Geometry check sheet. Reference: the model listing, model coordinates, mm. A direction names the side the tool comes from. Round coordinates to 2 decimals unless told otherwise and drop trailing zeros. Write each loop counter-clockwise with the first axis right and the second up, starting at its lowest first coordinate (ties: lowest second). Pieces come first, ordered by that corner, then holes. Notation, with made-up numbers: M -22.5,-30 L 14.5,-30 A20 ccw 14.5,-25 Z; hole C -21.75,74.25 d4. An arc over 180 degrees is marked long. Use a Markdown table: item, result.
```python
from build123d import *

# Parameters (mm, degrees)
BOSS_EXTRUDE1_DEPTH = 1.651
SKETCH3_W           = 2.54
SKETCH3_H           = 1.694812446
SKETCH3_W_2         = 1.694812446
SKETCH3_H_2         = 2.54
BOSS_EXTRUDE2_DEPTH = 3.683
BOSS_EXTRUDE3_DEPTH = 1.27
BOSS_EXTRUDE4_DEPTH = 1.27
FILLET1_R           = 1.27
CHAMFER1_SIZE       = 0.508
FILLET2_R           = 0.254


with BuildPart() as part:
    # Sketch1 → Boss-Extrude1 (new body)
    with BuildSketch(Plane(origin=(0, 0, 0), x_dir=(1, 0, 0), z_dir=(0, 1, 0))):
        with BuildLine():
            Line((-7.62, 7.112), (-7.62, -7.112))
            ThreePointArc((-7.62, -7.112), (-7.471210245, -7.471210245), (-7.112, -7.62))
            Line((-7.112, -7.62), (7.112, -7.62))
            ThreePointArc((7.112, -7.62), (7.471210245, -7.471210245), (7.62, -7.112))
            Line((7.62, -7.112), (7.62, 7.112))
            ThreePointArc((7.62, 7.112), (7.471210245, 7.471210245), (7.112, 7.62))
            Line((7.112, 7.62), (-7.112, 7.62))
            ThreePointArc((-7.112, 7.62), (-7.471210245, 7.471210245), (-7.62, 7.112))
        make_face()
    extrude(amount=BOSS_EXTRUDE1_DEPTH)

    # Sketch3 → Boss-Extrude2 (add)
    with BuildSketch(Plane(origin=(0, 1.651, 0), x_dir=(1, 0, 0), z_dir=(0, 1, 0))):
        with Locations((0, 3.013059552)):
            Rectangle(SKETCH3_W, SKETCH3_H)
        with Locations((3.013059552, 0)):
            Rectangle(SKETCH3_W_2, SKETCH3_H_2)
        with Locations((0, -3.013059552)):
            Rectangle(SKETCH3_W, SKETCH3_H)
        with Locations((-3.013059552, 0)):
            Rectangle(SKETCH3_W_2, SKETCH3_H_2)
    extrude(amount=BOSS_EXTRUDE2_DEPTH)

    # Sketch4 → Boss-Extrude3 (add, symmetric)
    with BuildSketch(Plane.XY):
        with BuildLine():
            Line((-3.860465775, 5.334), (-4.251394799, 4.259931334))
            ThreePointArc((-4.251394799, 4.259931334), (-4.201247752, 3.879026697), (-3.860465775, 3.701626828))
            Line((-3.860465775, 3.701626828), (-3.860465775, 5.334))
        make_face()
        with BuildLine():
            Line((3.860465775, 5.334), (4.251394799, 4.259931334))
            ThreePointArc((4.251394799, 4.259931334), (4.201247752, 3.879026697), (3.860465775, 3.701626828))
            Line((3.860465775, 3.701626828), (3.860465775, 5.334))
        make_face()
    extrude(amount=BOSS_EXTRUDE3_DEPTH, both=True)

    # Sketch5 → Boss-Extrude4 (add, symmetric)
    with BuildSketch(Plane(origin=(0, 0, 0), x_dir=(0, 0, -1), z_dir=(1, 0, 0))):
        with BuildLine():
            Line((-3.860465775, 5.334), (-4.251394799, 4.259931334))
            ThreePointArc((-4.251394799, 4.259931334), (-4.201512131, 3.878082751), (-3.860465775, 3.699242027))
            Line((-3.860465775, 3.699242027), (-3.860465775, 5.334))
        make_face()
        with BuildLine():
            Line((3.860465775, 5.334), (4.251394799, 4.259931334))
            ThreePointArc((4.251394799, 4.259931334), (4.201512131, 3.878082751), (3.860465775, 3.699242027))
            Line((3.860465775, 3.699242027), (3.860465775, 5.334))
        make_face()
    extrude(amount=BOSS_EXTRUDE4_DEPTH, both=True)

    # Fillet1
    fillet1_edges = [part.edges().sort_by_distance(p)[0] for p in [
        (0, 5.334, -3.860465775),
        (3.860465775, 5.334, 0),
        (0, 5.334, 3.860465775),
        (-3.860465775, 5.334, 0),
    ]]
    fillet(fillet1_edges, radius=FILLET1_R)

    # Chamfer1
    chamfer1_edges = [part.edges().sort_by_distance(p)[0] for p in [
        (7.471210245, 1.651, 7.471210245),
        (7.62, 1.651, 0),
        (7.471210245, 1.651, -7.471210245),
        (0, 1.651, -7.62),
        (-7.471210245, 1.651, -7.471210245),
        (-7.62, 1.651, 0),
        (-7.471210245, 1.651, 7.471210245),
        (0, 1.651, 7.62),
    ]]
    chamfer(chamfer1_edges, length=CHAMFER1_SIZE - 0.0001)  # a hair under: the kernel refuses the full size

    # Fillet2
    fillet2_edges = [part.edges().sort_by_distance(p)[0] for p in [
        (0, 0, 7.62),
        (-7.471210245, 0, 7.471210245),
        (-7.62, 0, 0),
        (-7.471210245, 0, -7.471210245),
        (0, 0, -7.62),
        (7.471210245, 0, -7.471210245),
        (7.62, 0, 0),
        (7.471210245, 0, 7.471210245),
    ]]
    fillet(fillet2_edges, radius=FILLET2_R)


solid = part.part
```
Item 1: Cross-section at B-B, the plane y = 2.5. Record the cut outline in (x, z), and give its area (3 significant figures).
Outcome:
| item | result |
|---|---|
| outline | M -3.86,-1.27 L -2.17,-1.27 L -2.17,1.27 L -3.86,1.27 Z; M -1.27,-3.86 L 1.27,-3.86 L 1.27,-2.17 L -1.27,-2.17 Z; M -1.27,2.17 L 1.27,2.17 L 1.27,3.86 L -1.27,3.86 Z; M 2.17,-1.27 L 3.86,-1.27 L 3.86,1.27 L 2.17,1.27 Z |
| area | 17.2 mm2 |
Item 2: Go/stop test with flat-tipped pins: pin 1 (1.7 mm diameter, centred on y = 3, z = -3.5, fed in from +X); pin 2 (3 mm diameter, centred on y = 4, z = -0.5, fed in from -X); pin 3 (0.8 mm diameter, centred on y = 3.5, z = 0, fed in from +X) (3 decimals); pin 4 (2 mm diameter, centred on x = 2, z = -5.5, fed in from -Y). Record where each tip stops, or that it passes through.
Outcome:
| item | result |
|---|---|
| pin 1 | stops at x = 1.27 |
| pin 2 | stops at x = -4.28 |
| pin 3 | stops at x = 4.215 |
| pin 4 | stops at y = 0 |
Item 3: Access from +Z, -Z, +X, -X, +Y, -Y to the whole of each face (thin tool, end or side, straight path). Record for faces 1 (the face through (0, 3, -3.86)), 2 (the face through (3, 4, 1.27)), 3 (the face through (3, 4, -1.27)).
Outcome:
| item | result |
|---|---|
| face 1 | -Z, +X, -X |
| face 2 | +Z, +X, -X, +Y |
| face 3 | -Z, +X, -X, +Y |
Item 4: Mould release check, pull along Y, two halves, no side actions. Record for faces 4 (the face through (0, 3, 2.166)), 5 (the face through (0, 5.334, 2.6)), 6 (the face through (0, 3, 3.86)): +Y half, -Y half, draft (parallel to the pull), parting line (faces both ways), or undercut.
Outcome:
| item | result |
|---|---|
| face 4 | draft |
| face 5 | +Y half |
| face 6 | undercut |
Item 5: Material ranges on line 1 along X through (y, z) = (2.05, -0.25); line 2 along Z through (x, y) = (-1, 4.25); line 3 along Y through (x, z) = (-5.25, -5.5), recorded low to high. Write a range as from..to.
Outcome:
| item | result |
|---|---|
| line 1 | x = -3.86..-2.17, 2.17..3.86 |
| line 2 | z = -4.25..-2.17, 2.17..4.25 |
| line 3 | y = 0..1.65 |
Item 6: Cross-section at C-C, the plane z = 1.5. Record the cut outline in (x, y), and give its area (3 significant figures).
Outcome:
| item | result |
|---|---|
| outline | M -7.62,0.25 A0.25 ccw -7.37,0 L 7.37,0 A0.25 ccw 7.62,0.25 L 7.62,1.14 L 7.11,1.65 L -7.11,1.65 L -7.62,1.14 Z |
| area | 24.9 mm2 |
Item 7: Cross-section at D-D, the plane z = -2.5. Record the cut outline in (x, y).
Outcome:
| item | result |
|---|---|
| outline | M -7.62,0.25 A0.25 ccw -7.37,0 L 7.37,0 A0.25 ccw 7.62,0.25 L 7.62,1.14 L 7.11,1.65 L 1.27,1.65 L 1.27,5.33 L -1.27,5.33 L -1.27,1.65 L -7.11,1.65 L -7.62,1.14 Z |
Item 8: Cross-section at A-A, the plane x = 2.5. Record the cut outline in (y, z), and give its area (3 significant figures).
Outcome:
| item | result |
|---|---|
| outline | M 0,-7.37 A0.25 ccw 0.25,-7.62 L 1.14,-7.62 L 1.65,-7.11 L 1.65,-1.27 L 5.33,-1.27 L 5.33,1.27 L 1.65,1.27 L 1.65,7.11 L 1.14,7.62 L 0.25,7.62 A0.25 ccw 0,7.37 Z |
| area | 34.2 mm2 |
